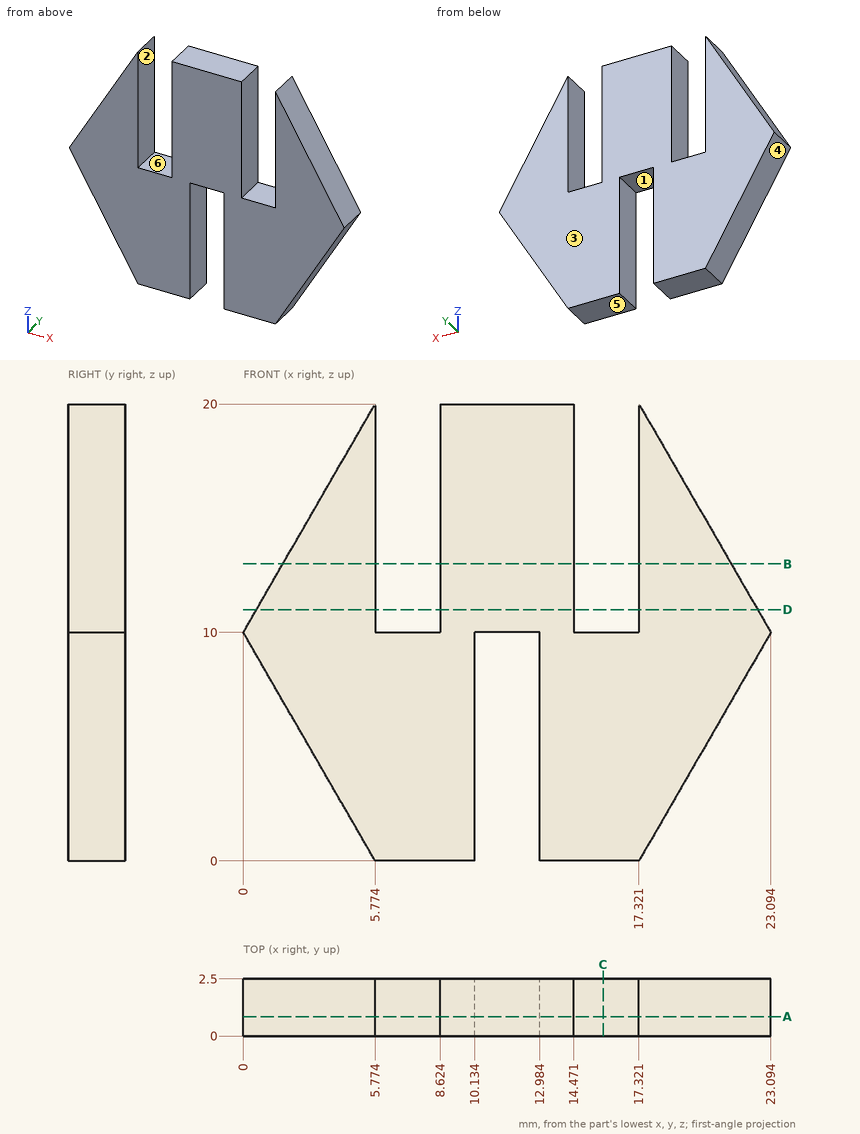
The drawing under review shows one solid part. Ordinate dimensions are in mm from its lowest x, y, z. A direction names the side the tool comes from. Round coordinates to 2 decimals unless told otherwise and drop trailing zeros. Loops run counter-clockwise (first coordinate to the right, second up) from the corner with the lowest first, then second, coordinate; pieces in that order, holes last. Notation, with made-up numbers: (80.25, -20.5) - (84.25, -20.5) arc R31 ccw to (84.25, 18.5) - close; hole circle Ø9 at (49.5, 42.25). An arc over 180 degrees is marked (long way). One line per item, written item: value. Start each with the question number.
1) Consider section D-D on z = 11. Give the boundary of the cut face in (x, y).
2) Insertion check: pin 1 Ø0.8 at (y, z) = (1.5, 14) entering from +X (1 decimal); pin 2 Ø0.8 at (x, y) = (11, 1) entering from -Z; pin 3 Ø1.2 at (x, y) = (15.5, 1.5) entering from +Z. Each pin has a flat end and moves straight along its axis. Give the tip position at first contact, or say it passes through.
3) Consider section C-C on x = 15.75. Give the boundary of the cut face in (y, z).
4) Consider section A-A on y = 0.85. Give the boundary of the cut face in (x, z) (1 decimal), then the cut area to 3 significant figures.
5) To check wall thickness, follow L1, parallel to X at y = 0.75, z = 18.25 (1 decimal); L2, parallel to X at y = 1.75, z = 13.5 (1 decimal); L3, parallel to Z at x = 10.5, y = 1.8. State the ranges of each line that lie inside material, in increasing order. Write a range as from..to.
6) Draft analysis for pull direction X (two halves, no side actions). For the marked faces 4, 5 and 6, state which applies: +X half, -X half, draft (parallel to the pull), parting line (faces both ways), or undercut.
7) Consider section B-B on z = 13. Give the boundary of the cut face in (x, y).
8) For the marked faces 1, 2 and 3, list the 3-axis set-ups (+Z, -Z, +X, -X, +Y, -Y) from which the entire face can be reached by the end or side of a thin tool; tool diameter is ignored.
Reported:
1. outline: (0.58, 0) - (5.77, 0) - (5.77, 2.5) - (0.58, 2.5) - close; (8.62, 0) - (14.47, 0) - (14.47, 2.5) - (8.62, 2.5) - close; (17.32, 0) - (22.52, 0) - (22.52, 2.5) - (17.32, 2.5) - close
2. pin 1: stops at x = 21
2. pin 2: stops at z = 10
2. pin 3: stops at z = 10
3. outline: (0, 0) - (2.5, 0) - (2.5, 10) - (0, 10) - close
4. outline: (0, 10) - (5.8, 0) - (10.1, 0) - (10.1, 10) - (13, 10) - (13, 0) - (17.3, 0) - (23.1, 10) - (17.3, 20) - (17.3, 10) - (14.5, 10) - (14.5, 20) - (8.6, 20) - (8.6, 10) - (5.8, 10) - (5.8, 20) - close
4. area: 261 mm^2
5. L1: x = 4.8..5.8, 8.6..14.5, 17.3..18.3
5. L2: x = 2..5.8, 8.6..14.5, 17.3..21.1
5. L3: z = 10..20
6. face 4: -X half
6. face 5: draft
6. face 6: undercut
7. outline: (1.73, 0) - (5.77, 0) - (5.77, 2.5) - (1.73, 2.5) - close; (8.62, 0) - (14.47, 0) - (14.47, 2.5) - (8.62, 2.5) - close; (17.32, 0) - (21.36, 0) - (21.36, 2.5) - (17.32, 2.5) - close
8. face 1: -Z, +Y, -Y
8. face 2: +Z, +Y, -Y
8. face 3: +Z, -Z, +X, -X, +Y
